Work out the finished part from the listing and answer in its coordinate system (mm). Coordinates: 2 decimals unless noted, no trailing zeros. Order: outer loops, then holes, each group sorted by start corner. A loop starts at its lowest first (then second) coordinate and runs counter-clockwise, first axis right, second up.
```python
from build123d import *

# Parameters (mm, degrees)
SKETCH_1_W          = 220
SKETCH_1_H          = 123.55
EXTRUDE_1_DEPTH     = 1.5
SKETCH_2_R          = 18.5
SKETCH_2_R_2        = 1.5
CUT_EXTRUDE_1_DEPTH = 10


with BuildPart() as part:
    # 草图1 → 凸台-拉伸1 (new body)
    with BuildSketch(Plane(origin=(0, 0, 0), x_dir=(1, 0, 0), z_dir=(0, 1, 0))):
        with Locations((44.295012832, -17.457747405)):
            Rectangle(SKETCH_1_W, SKETCH_1_H)
    extrude(amount=EXTRUDE_1_DEPTH)

    # 草图2 → 切除-拉伸1 (cut)
    with BuildSketch(Plane(origin=(0, 1.5, 0), x_dir=(1, 0, 0), z_dir=(0, 1, 0))):
        with Locations(Location((-31.57031265, -12.457747405, 0), (0, 0, 270))):
            Circle(SKETCH_2_R)
        with Locations(Location((-47.67031265, 3.642252595, 0), (0, 0, 270))):
            Circle(SKETCH_2_R_2)
        with Locations(Location((-47.67031265, -28.557747405, 0), (0, 0, 270))):
            Circle(SKETCH_2_R_2)
        with Locations(Location((149.295012832, -69.232747405, 0), (0, 0, 270))):
            Circle(SKETCH_2_R_2)
        with Locations(Location((44.295012832, -69.232747405, 0), (0, 0, 270))):
            Circle(SKETCH_2_R_2)
        with Locations(Location((-60.704987168, -69.232747405, 0), (0, 0, 270))):
            Circle(SKETCH_2_R_2)
        with Locations(Location((44.295012832, -49.232747405, 0), (0, 0, 270))):
            Circle(SKETCH_2_R_2)
        with Locations(Location((-60.704987168, -49.232747405, 0), (0, 0, 270))):
            Circle(SKETCH_2_R_2)
        with Locations(Location((149.295012832, -49.232747405, 0), (0, 0, 270))):
            Circle(SKETCH_2_R_2)
        with Locations(Location((149.295012832, 14.317252595, 0), (0, 0, 270))):
            Circle(SKETCH_2_R_2)
        with Locations(Location((-60.704987168, 14.317252595, 0), (0, 0, 270))):
            Circle(SKETCH_2_R_2)
        with Locations(Location((44.295012832, 14.317252595, 0), (0, 0, 270))):
            Circle(SKETCH_2_R_2)
        with Locations(Location((-60.704987168, 34.317252595, 0), (0, 0, 270))):
            Circle(SKETCH_2_R_2)
        with Locations(Location((44.295012832, 34.317252595, 0), (0, 0, 270))):
            Circle(SKETCH_2_R_2)
        with Locations(Location((149.295012832, 34.317252595, 0), (0, 0, 270))):
            Circle(SKETCH_2_R_2)
        with Locations(Location((149.295012832, -29.232747405, 0), (0, 0, 270))):
            Circle(SKETCH_2_R_2)
        with Locations(Location((44.295012832, -29.232747405, 0), (0, 0, 270))):
            Circle(SKETCH_2_R_2)
        with Locations(Location((-60.704987168, -29.232747405, 0), (0, 0, 270))):
            Circle(SKETCH_2_R_2)
        with Locations(Location((149.295012832, -5.682747405, 0), (0, 0, 270))):
            Circle(SKETCH_2_R_2)
        with Locations(Location((44.295012832, -5.682747405, 0), (0, 0, 270))):
            Circle(SKETCH_2_R_2)
        with Locations(Location((-60.704987168, -5.682747405, 0), (0, 0, 270))):
            Circle(SKETCH_2_R_2)
        with Locations(Location((-15.47031265, 3.642252595, 0), (0, 0, 270))):
            Circle(SKETCH_2_R_2)
        with Locations(Location((-15.47031265, -28.557747405, 0), (0, 0, 270))):
            Circle(SKETCH_2_R_2)
    extrude(amount=-CUT_EXTRUDE_1_DEPTH, mode=Mode.SUBTRACT)


solid = part.part
```
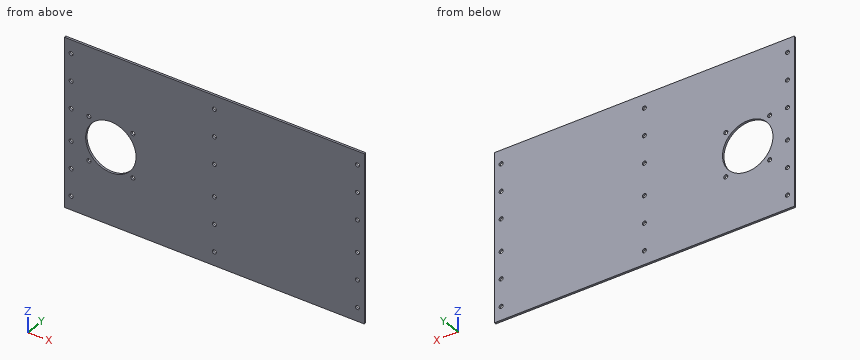
1. The part is cut by section B-B (y = 0.55). Count the separate pieces of the cut face and the enclosed holes in it, plus the area to 3 significant figures.
2. Consider probe 1 along Z at (x, y) = (-47.5, 0.9); probe 2 along X at (y, z) = (0.1, 11.5); probe 3 along X at (y, z) = (0.7, -35). Determine where each line is inside the solid, lowest interval first.
3. The part is cut by section A-A (z = 12). Determine the outline of the cut face in (x, y).
Worked out:
1. separate pieces: 1
1. enclosed holes: 23
1. area: 26,000 mm2
2. probe 1: z = -44.32 to -5.13, -2.15 to 3.05, 21.86 to 27.07, 30.05 to 79.23
2. probe 2: x = -65.7 to -50.05, -13.1 to 154.3
2. probe 3: x = -65.7 to -62.04, -59.37 to 42.96, 45.63 to 147.96, 150.63 to 154.3
3. outline: (-65.7, 0) - (-50.06, 0) - (-50.06, 1.5) - (-65.7, 1.5) - close; (-13.08, 0) - (154.3, 0) - (154.3, 1.5) - (-13.08, 1.5) - close
